from build123d import *

# Parameters (mm, degrees)
CROQUIS1_W              = 30
CROQUIS1_H              = 126
SALIENTE_EXTRUIR1_DEPTH = 4
CROQUIS3_R              = 2
CORTAR_EXTRUIR2_DEPTH   = 5
CROQUIS8_R              = 2.55
CORTAR_EXTRUIR3_DEPTH   = 5
CROQUIS21_W             = 5
CROQUIS21_H             = 23
SALIENTE_EXTRUIR2_DEPTH = 4
CORTAR_EXTRUIR16_DEPTH  = 5
CROQUIS11_R             = 1.575
CORTAR_EXTRUIR8_DEPTH   = 5
CROQUIS15_R             = 1.575
CORTAR_EXTRUIR11_DEPTH  = 5
CHAFL_N2_SIZE           = 3
CROQUIS19_R             = 3.5
CORTAR_EXTRUIR13_DEPTH  = 1.9
CROQUIS20_R             = 3.05
CORTAR_EXTRUIR14_DEPTH  = 2
CROQUIS24_W             = 35
CROQUIS24_H             = 2.2
SALIENTE_EXTRUIR3_DEPTH = 4


with BuildPart() as part:
    # Croquis1 → Saliente-Extruir1 (new body)
    with BuildSketch(Plane(origin=(0, 0, 0), x_dir=(0, 0, -1), z_dir=(1, 0, 0))):
        Rectangle(CROQUIS1_W, CROQUIS1_H)
    extrude(amount=SALIENTE_EXTRUIR1_DEPTH)

    # Croquis3 → Cortar-Extruir2 (cut, through all)
    with BuildSketch(Plane(origin=(4, 0, 0), x_dir=(0, 0, -1), z_dir=(1, 0, 0))):
        with Locations((-10, 10.1)):
            Circle(CROQUIS3_R)
        with Locations((10, 10.1)):
            Circle(CROQUIS3_R)
        with Locations((-10, -9.9)):
            Circle(CROQUIS3_R)
        with Locations((10, -9.9)):
            Circle(CROQUIS3_R)
    extrude(amount=-CORTAR_EXTRUIR2_DEPTH, mode=Mode.SUBTRACT)

    # Croquis8 → Cortar-Extruir3 (cut, through all)
    with BuildSketch(Plane.ZY):
        with Locations((0, 45.75)):
            Circle(CROQUIS8_R)
    extrude(amount=-CORTAR_EXTRUIR3_DEPTH, mode=Mode.SUBTRACT)

    # Croquis21 → Saliente-Extruir2 (add)
    with BuildSketch(Plane.ZY):
        with Locations((17.5, -51.5)):
            Rectangle(CROQUIS21_W, CROQUIS21_H)
    extrude(amount=-SALIENTE_EXTRUIR2_DEPTH)

    # Croquis23 → Cortar-Extruir16 (cut, through all)
    with BuildSketch(Plane(origin=(4, 0, 0), x_dir=(0, 0, -1), z_dir=(1, 0, 0))):
        with BuildLine():
            Line((-15.240890395, -43.96), (-15.240890395, -49.96))
            ThreePointArc((-15.240890395, -49.96), (-16.790890395, -51.51), (-18.340890395, -49.96))
            Line((-18.340890395, -49.96), (-18.340890395, -43.96))
            ThreePointArc((-18.340890395, -43.96), (-16.790890395, -42.41), (-15.240890395, -43.96))
        make_face()
        with BuildLine():
            Line((-3.857181896, -55.343708499), (-3.857181896, -61.343708499))
            ThreePointArc((-3.857181896, -61.343708499), (-5.407181896, -62.893708499), (-6.957181896, -61.343708499))
            Line((-6.957181896, -61.343708499), (-6.957181896, -55.343708499))
            ThreePointArc((-6.957181896, -55.343708499), (-5.407181896, -53.793708499), (-3.857181896, -55.343708499))
        make_face()
    extrude(amount=-CORTAR_EXTRUIR16_DEPTH, mode=Mode.SUBTRACT)

    # Croquis11 → Cortar-Extruir8 (cut, through all)
    with BuildSketch(Plane(origin=(4, 0, 0), x_dir=(0, 0, -1), z_dir=(1, 0, 0))):
        with Locations((2, 34.75)):
            Circle(CROQUIS11_R)
        with Locations((2, 24.75)):
            Circle(CROQUIS11_R)
    extrude(amount=-CORTAR_EXTRUIR8_DEPTH, mode=Mode.SUBTRACT)

    # Croquis15 → Cortar-Extruir11 (cut, through all)
    with BuildSketch(Plane(origin=(4, 0, 0), x_dir=(0, 0, -1), z_dir=(1, 0, 0))):
        with Locations((-10.4, 57.45)):
            Circle(CROQUIS15_R)
        with Locations((10.4, 57.45)):
            Circle(CROQUIS15_R)
        with Locations((-10.4, 25.1)):
            Circle(CROQUIS15_R)
        with Locations((10.4, 25.1)):
            Circle(CROQUIS15_R)
    extrude(amount=-CORTAR_EXTRUIR11_DEPTH, mode=Mode.SUBTRACT)

    # Chaflán2
    chafl_n2_edges = [part.edges().sort_by_distance(p)[0] for p in [
        (2, 63, -15),
        (2, 63, 15),
    ]]
    chamfer(chafl_n2_edges, length=CHAFL_N2_SIZE)

    # Croquis19 → Cortar-Extruir13 (cut)
    with BuildSketch(Plane.ZY):
        with Locations((-2, 24.75)):
            Circle(CROQUIS19_R)
        with Locations((-2, 34.75)):
            Circle(CROQUIS19_R)
    extrude(amount=-CORTAR_EXTRUIR13_DEPTH, mode=Mode.SUBTRACT)

    # Croquis20 → Cortar-Extruir14 (cut)
    with BuildSketch(Plane(origin=(4, 0, 0), x_dir=(0, 0, -1), z_dir=(1, 0, 0))):
        with Locations((-10.4, 57.45)):
            Circle(CROQUIS20_R)
        with Locations((10.4, 57.45)):
            Circle(CROQUIS20_R)
        with Locations((10.4, 25.1)):
            Circle(CROQUIS20_R)
        with Locations((-10.4, 25.1)):
            Circle(CROQUIS20_R)
    extrude(amount=-CORTAR_EXTRUIR14_DEPTH, mode=Mode.SUBTRACT)

    # Croquis24 → Saliente-Extruir3 (add)
    with BuildSketch(Plane(origin=(4, 0, 0), x_dir=(0, 0, -1), z_dir=(1, 0, 0))):
        with Locations((-2.5, -64.1)):
            Rectangle(CROQUIS24_W, CROQUIS24_H)
    extrude(amount=-SALIENTE_EXTRUIR3_DEPTH)


solid = part.part
Check sheet for the modelled part. Datum: model origin and axes. Units: mm. A direction names the side the tool comes from. Give positions to 0.01 mm unless a question says otherwise; leave off trailing zeros. Write each loop counter-clockwise with the first axis right and the second up, starting at its lowest first coordinate (ties: lowest second). Pieces come first, ordered by that corner, then holes. Notation, with made-up numbers: (8.5, 39.5) -> (65.5, 39.5) arc R19 ccw to (65.5, 55.5) -> close; hole circle Ø7 at (15, 84.25). An arc over 180 degrees is marked (long way). One line per item, written item: value. Start each with the question number.
Item 1: Material ranges on probe 1 along Z at (x, y) = (2.6, 10); probe 2 along Y at (x, z) = (2.75, 10); probe 3 along Y at (x, z) = (0.9, -10.4) (3 decimals), recorded low to high. Write a range as from..to.
Item 2: Section check B-B on x = 2.8. State how many separate pieces and enclosed holes the cut face has, then the cut area to 3 significant figures.
Item 3: Section check C-C on z = 10.4. Record the cut outline in (x, y) (3 decimals), then the cut area to 3 significant figures.
Item 4: Gauge pin test, flat ends, axial feed: pin 1 (3.5 mm diameter, centred on y = 10.1, z = 10, fed in from +X); pin 2 (3.5 mm diameter, centred on y = 57.45, z = 10.4, fed in from +X). Record the tip position at first contact, or that the pin passes through.
Item 5: Tool access check on faces 1 (the flat face through (2, 24, 9)), 2 (the flat face through (2, -40, 17)), 3 (the cylindrical face through (2.03, -51.51, 16.76)). Record the directions out of +Z, -Z, +X, -X, +Y, -Y that give a thin tool (end or side, any length) a straight path to the whole face; none if there is none.
Item 6: Section check A-A on y = 57.45. Record the cut outline in (x, z) (3 decimals), then the cut area to 3 significant figures.
Item 7: Section check D-D on z = -10. Record the cut outline in (x, y).
Results list:
1. probe 1: -15..-12, -8..8, 12..15
1. probe 2: -65.2..-11.9, -7.9..8.1, 12.1..22.08, 28.12..54.43, 60.47..63
1. probe 3: -65.2..-11.86, -7.94..8.14, 12.06..23.525, 26.675..55.875, 59.025..63
2. separate pieces: 1
2. enclosed holes: 13
2. area: 3,710 mm²
3. outline: (0, -65.2) -> (4, -65.2) -> (4, -11.86) -> (0, -11.86) -> close; (0, -7.94) -> (4, -7.94) -> (4, 8.14) -> (0, 8.14) -> close; (0, 12.06) -> (4, 12.06) -> (4, 22.05) -> (2, 22.05) -> (2, 23.525) -> (0, 23.525) -> close; (0, 26.675) -> (2, 26.675) -> (2, 28.15) -> (4, 28.15) -> (4, 54.4) -> (2, 54.4) -> (2, 55.875) -> (0, 55.875) -> close; (0, 59.025) -> (2, 59.025) -> (2, 60.5) -> (4, 60.5) -> (4, 63) -> (0, 63) -> close
3. area: 444 mm²
4. pin 1: through
4. pin 2: x = 2
5. face 1: +X
5. face 2: +Z, +X, -X, +Y
5. face 3: +X, -X
6. outline: (0, -15) -> (4, -15) -> (4, -13.45) -> (2, -13.45) -> (2, -11.975) -> (0, -11.975) -> close; (0, -8.825) -> (2, -8.825) -> (2, -7.35) -> (4, -7.35) -> (4, 7.35) -> (2, 7.35) -> (2, 8.825) -> (0, 8.825) -> close; (0, 11.975) -> (2, 11.975) -> (2, 13.45) -> (4, 13.45) -> (4, 15) -> (0, 15) -> close
6. area: 83.0 mm²
7. outline: (0, -65.2) -> (4, -65.2) -> (4, -11.9) -> (0, -11.9) -> close; (0, -7.9) -> (4, -7.9) -> (4, 8.1) -> (0, 8.1) -> close; (0, 12.1) -> (4, 12.1) -> (4, 22.08) -> (2, 22.08) -> (2, 23.58) -> (0, 23.58) -> close; (0, 26.62) -> (2, 26.62) -> (2, 28.12) -> (4, 28.12) -> (4, 54.43) -> (2, 54.43) -> (2, 55.93) -> (0, 55.93) -> close; (0, 58.97) -> (2, 58.97) -> (2, 60.47) -> (4, 60.47) -> (4, 63) -> (0, 63) -> close
